```python
from build123d import *

# Parameters (mm, degrees)
BOSS_EXTRUDE1_DEPTH = 40
FILLET1_SIZE        = 15
FILLET1_SIZE_2      = 4
FILLET2_SIZE        = 15
FILLET2_SIZE_2      = 4
FILLET3_SIZE        = 15
FILLET3_SIZE_2      = 4
FILLET4_SIZE        = 15
FILLET4_SIZE_2      = 4
FILLET5_R           = 3
FILLET6_R           = 0.45
FILLET8_R           = 7
FILLET9_R           = 3
FILLET10_R          = 4
CUT_EXTRUDE1_DEPTH  = 147.245106811
FILLET11_R          = 4


with BuildPart() as part:
    # Sketch1 → Boss-Extrude1 (new body)
    with BuildSketch(Plane.XY):
        with BuildLine():
            ThreePointArc((6.77692336, 14.493905953), (-5.565334282, 14.795328723), (-14.153654854, 5.926116291))
            Line((-14.153654854, 5.926116291), (-53.584656115, -100))
            Line((-53.584656115, -100), (-74.316504114, -100))
            Line((-74.316504114, -100), (-74.316504114, -105))
            Line((-74.316504114, -105), (-24.316504114, -105))
            Line((-24.316504114, -105), (-24.316504114, -100))
            Line((-24.316504114, -100), (-45.048352113, -100))
            Line((-45.048352113, -100), (-6.656264884, 3.135212559))
            ThreePointArc((-6.656264884, 3.135212559), (-2.534671543, 7.39160781), (3.38846168, 7.246952976))
            Line((3.38846168, 7.246952976), (0, 0))
            Line((0, 0), (37.593568565, -17.577644966))
            Line((37.593568565, -17.577644966), (35.899337725, -21.201121454))
            Line((35.899337725, -21.201121454), (45.863898068, -25.860256264))
            Line((45.863898068, -25.860256264), (49.252359748, -18.613303288))
            ThreePointArc((49.252359748, -18.613303288), (48.287736924, -15.954449623), (45.62888326, -16.919072448))
            Line((45.62888326, -16.919072448), (43.93465242, -20.542548936))
            Line((43.93465242, -20.542548936), (41.217045053, -19.271875806))
            Line((41.217045053, -19.271875806), (42.911275893, -15.648399317))
            Line((42.911275893, -15.648399317), (5.317707328, 1.929245648))
            Line((5.317707328, 1.929245648), (12.094630689, 16.423151601))
            Line((12.094630689, 16.423151601), (49.688199254, -1.154493365))
            Line((49.688199254, -1.154493365), (51.382430094, 2.468983124))
            Line((51.382430094, 2.468983124), (54.10003746, 1.198309994))
            Line((54.10003746, 1.198309994), (52.40580662, -2.425166495))
            ThreePointArc((52.40580662, -2.425166495), (53.370429444, -5.084020159), (56.029283108, -4.119397335))
            Line((56.029283108, -4.119397335), (59.417744788, 3.127555642))
            Line((59.417744788, 3.127555642), (49.453184446, 7.786690452))
            Line((49.453184446, 7.786690452), (47.758953606, 4.163213964))
            Line((47.758953606, 4.163213964), (10.16538504, 21.740858929))
            Line((10.16538504, 21.740858929), (6.77692336, 14.493905953))
        make_face()
    extrude(amount=BOSS_EXTRUDE1_DEPTH)

    # Fillet1
    # an asymmetric fillet: 15, 4 mm, written as the material it takes off along each edge
    with BuildSketch(Plane(origin=(49.688199254, -1.154493365, -37.5), x_dir=(-0.9058691220518403, 0.42355771001485515, 0), z_dir=(0, 0, 1))) as fillet1_piece_1:
        with BuildLine():
            Bezier((FILLET1_SIZE, 0), (0, 0), (0, -FILLET1_SIZE_2), weights=[1, 0.707106781, 1])
            Line((0, -FILLET1_SIZE_2), (0, 0))
            Line((0, 0), (FILLET1_SIZE, 0))
        make_face()
    extrude(amount=115, mode=Mode.SUBTRACT)

    # Fillet2
    # an asymmetric fillet: 15, 4 mm, written as the material it adds along each edge
    with BuildSketch(Plane(origin=(47.758953606, 4.163213964, 0), x_dir=(-0.9058691220518406, 0.42355771001485454, 0), z_dir=(0, 0, 1))) as fillet2_piece_1:
        with BuildLine():
            Bezier((FILLET2_SIZE, 0), (0, 0), (0, -FILLET2_SIZE_2), weights=[1, 0.707106781, 1])
            Line((0, -FILLET2_SIZE_2), (0, 0))
            Line((0, 0), (FILLET2_SIZE, 0))
        make_face()
    extrude(amount=40)

    # Fillet3
    # an asymmetric fillet: 15, 4 mm, written as the material it takes off along each edge
    with BuildSketch(Plane(origin=(42.911275893, -15.648399317, -37.5), x_dir=(-0.9058691220518403, 0.4235577100148549, 0), z_dir=(0, 0, 1))) as fillet3_piece_1:
        with BuildLine():
            Bezier((FILLET3_SIZE, 0), (0, 0), (0, FILLET3_SIZE_2), weights=[1, 0.707106781, 1])
            Line((0, FILLET3_SIZE_2), (0, 0))
            Line((0, 0), (FILLET3_SIZE, 0))
        make_face()
    extrude(amount=115, mode=Mode.SUBTRACT)

    # Fillet4
    # an asymmetric fillet: 15, 4 mm, written as the material it adds along each edge
    with BuildSketch(Plane(origin=(37.593568565, -17.577644966, 0), x_dir=(-0.9058691220518404, 0.42355771001485476, 0), z_dir=(0, 0, 1))) as fillet4_piece_1:
        with BuildLine():
            Bezier((FILLET4_SIZE, 0), (0, 0), (0, FILLET4_SIZE_2), weights=[1, 0.707106781, 1])
            Line((0, FILLET4_SIZE_2), (0, 0))
            Line((0, 0), (FILLET4_SIZE, 0))
        make_face()
    extrude(amount=40)

    # Fillet5
    fillet5_edges = [part.edges().sort_by_distance(p)[0] for p in [
        (45.863898068, -25.860256264, 20),
        (59.417744788, 3.127555642, 20),
        (35.899337725, -21.201121454, 20),
        (49.453184446, 7.786690452, 20),
    ]]
    fillet(fillet5_edges, radius=FILLET5_R)

    # Fillet6
    fillet6_edges = [part.edges().sort_by_distance(p)[0] for p in [
        (41.217045053, -19.271875806, 20),
        (43.93465242, -20.542548936, 20),
        (51.382430094, 2.468983124, 20),
        (54.10003746, 1.198309994, 20),
    ]]
    fillet(fillet6_edges, radius=FILLET6_R)

    # Fillet8
    fillet8_edges = [part.edges().sort_by_distance(p)[0] for p in [
        (0, 0, 20),
        (10.16538504, 21.740858929, 20),
    ]]
    fillet(fillet8_edges, radius=FILLET8_R)

    # Fillet9
    fillet9_edges = [part.edges().sort_by_distance(p)[0] for p in [
        (5.317707328, 1.929245648, 20),
        (12.094630689, 16.423151601, 20),
    ]]
    fillet(fillet9_edges, radius=FILLET9_R)

    # Fillet10
    fillet10_edges = [part.edges().sort_by_distance(p)[0] for p in [
        (-45.048352113, -100, 20),
        (-53.584656115, -100, 20),
    ]]
    fillet(fillet10_edges, radius=FILLET10_R)

    # Sketch2 → Cut-Extrude1 (cut, through all)
    with BuildSketch(Plane(origin=(0, -100, 0), x_dir=(1, 0, 0), z_dir=(0, 1, 0))):
        with BuildLine():
            ThreePointArc((-68.09015603, -20), (-65.34015603, -22.75), (-62.59015603, -20))
            Line((-62.59015603, -20), (-68.09015603, -20))
        make_face()
        with BuildLine():
            Line((-68.09015603, -20), (-62.59015603, -20))
            ThreePointArc((-62.59015603, -20), (-65.34015603, -17.25), (-68.09015603, -20))
        make_face()
        with BuildLine():
            ThreePointArc((-34.553852028, -20), (-31.803852028, -22.75), (-29.053852028, -20))
            Line((-29.053852028, -20), (-34.553852028, -20))
        make_face()
        with BuildLine():
            Line((-34.553852028, -20), (-29.053852028, -20))
            ThreePointArc((-29.053852028, -20), (-31.803852028, -17.25), (-34.553852028, -20))
        make_face()
    extrude(amount=-CUT_EXTRUDE1_DEPTH, mode=Mode.SUBTRACT)

    # Fillet11
    fillet11_edges = [part.edges().sort_by_distance(p)[0] for p in [
        (-24.316504114, -100, 20),
        (-74.316504114, -100, 20),
    ]]
    fillet(fillet11_edges, radius=FILLET11_R)


solid = part.part
```
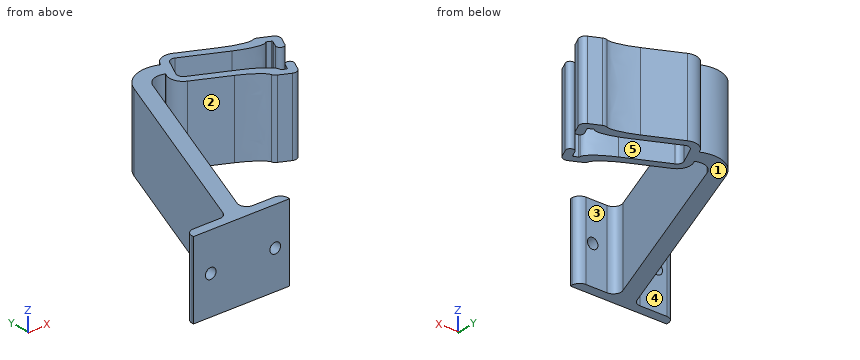
Can you work these out from the model? Positions are in its coordinate system, mm. Face numbers are marked on the shaded views. A direction names the side the tool comes from. Give positions to 0.01 mm unless a question says otherwise; leave off trailing zeros. Loops run counter-clockwise (first coordinate to the right, second up) from the corner with the lowest first, then second, coordinate; pieces in that order, holes last. Notation, with made-up numbers: M 61.5,77.5 L 110.5,77.5 A28 cw 110.5,103.5 Z; hole C -20.75,15 d4. An arc over 180 degrees is marked long. Use one line per item in the form item = value. Start each with the question number.
(1) I'm going to push flat-ended pins straight in: P1, Ø7, axis at x = -66, z = 25.5, coming from the +Y side; P2, Ø12, axis at y = -65, z = 22, coming from the -X side; P3, Ø3, axis at x = 21, z = 31.5, coming from the +Y side. Where does each tip first touch, or does it pass through?
(2) I want a section at B-B, the plane x = -1. Write out the boundary of the cut face in (y, z).
(3) On a 3-axis mill with a long thin cutter (end or side, diameter ignored), from which of +Z, -Z, +X, -X, +Y, -Y can I reach the whole of each face in a straight line? I mean the marked faces 1, 2, 3, 4 and 5. Say none if no direction works.
(4) Please list where these lines run through material, in increasing order: line 1 (X direction, y = -101.3, z = 20); line 2 (X direction, y = -103.05, z = 20); line 3 (Y direction, x = 22.5, z = 4).
(5) I want a section at C-C, the plane y = -26.5. Write out the boundary of the cut face in (x, z).
(6) I want a section at A-A, the plane z = 20. State how many separate pieces and enclosed holes the cut face has, and give its area (3 significant figures).
Worked out:
q1.P1 = -100
q1.P2 = -42.79
q1.P3 = 17.38
q2.outline = M 7.83,0 L 15.89,0 L 15.89,40 L 7.83,40 Z
q3.face_1 = -Z, +X, -X, +Y, -Y
q3.face_2 = +Z, -Z, -Y
q3.face_3 = +Z, -Z, +X
q3.face_4 = +Z, -Z, -X, +Y
q3.face_5 = +Z, -Z
q4.line_1 = -73.27 to -68.09, -62.59 to -34.55, -29.05 to -25.37
q4.line_2 = -74.2 to -68.09, -62.59 to -34.55, -29.05 to -24.43
q4.line_3 = -10.52 to -6.1, 11.56 to 15.97
q5.outline = M -26.22,0 L -17.69,0 L -17.69,40 L -26.22,40 Z
q6.separate_pieces = 3
q6.enclosed_holes = 0
q6.area = 1,780 mm²
